The figure shows three views and two pictorial views of one solid part (mm, origin at its lowest corner). Answer the questions. A direction names the side the tool comes from. Round coordinates to 2 decimals unless told otherwise and drop trailing zeros. Order: outer loops, then holes, each group sorted by start corner. A loop starts at its lowest first (then second) coordinate and runs counter-clockwise, first axis right, second up. Notation, with made-up numbers: (77, -31) -> (97, -31) arc R20 cw to (97, -13) -> close; hole circle Ø6 at (-26.5, -36.75). An arc over 180 degrees is marked (long way). Answer in a Markdown table with one row per item. Add a question column.
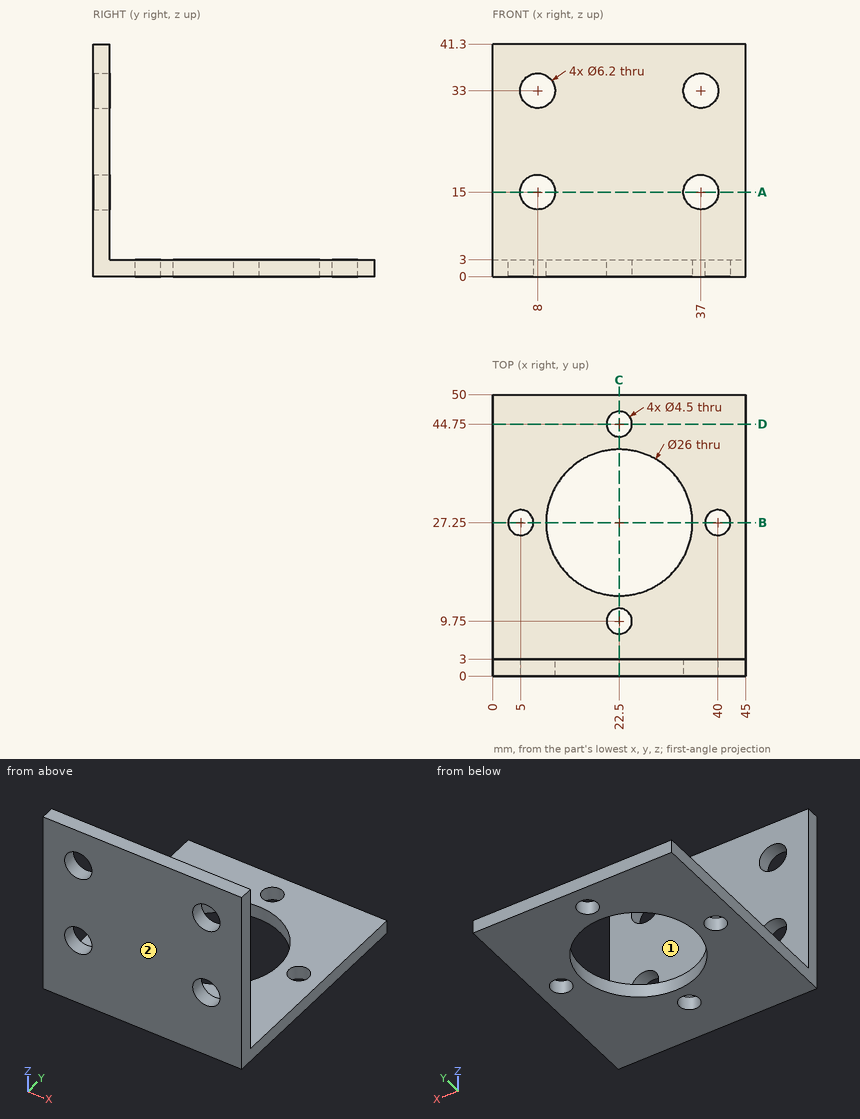
1. For the marked faces 1 and 2, determine the directions among +Z, -Z, +X, -X, +Y, -Y from which every point of the face is accessible in a straight line to the end or side of a thin tool.
2. Straight lines are drawn through the part: line 1 along Z through (x, y) = (8, 1); line 2 along X through (y, z) = (27, 2); line 3 along Y through (x, z) = (40, 1). For each, find the intervals that lie inside material, in ascending order.
3. The part is cut by section D-D (y = 44.75). Give the vertices of the cut face in (x, z).
4. The part is cut by section B-B (y = 27.25). Give the vertices of the cut face in (x, z), then the cut area to 3 significant figures.
5. The part is cut by section A-A (z = 15). Give the vertices of the cut face in (x, y).
6. Each of these flat-tipped pins is pushed along its axis until it touches: pin 1 (4 mm diameter, centred on y = 33.5, z = 5.5, fed in from -X); pin 2 (5 mm diameter, centred on x = 22.5, y = 9.75, fed in from -Z); pin 3 (19 mm diameter, centred on x = 12.5, z = 16, fed in from +Y); pin 4 (10 mm diameter, centred on x = 10, y = 43.5, fed in from +Z). Where does it stop, or does it pass through?
7. The part is cut by section C-C (x = 22.5). Give the vertices of the cut face in (y, z), then the cut area to 3 significant figures.
Report:
| question | item | result |
|---|---|---|
| 1 | face 1 | +Z, +X, -X, +Y |
| 1 | face 2 | +Z, -Z, +X, -X, -Y |
| 2 | line 1 | z = 0 to 11.9, 18.1 to 29.9, 36.1 to 41.3 |
| 2 | line 2 | x = 0 to 2.76, 7.24 to 9.5, 35.5 to 37.76, 42.24 to 45 |
| 2 | line 3 | y = 0 to 25, 29.5 to 50 |
| 3 | outline | (0, 0) -> (20.25, 0) -> (20.25, 3) -> (0, 3) -> close; (24.75, 0) -> (45, 0) -> (45, 3) -> (24.75, 3) -> close |
| 4 | outline | (0, 0) -> (2.75, 0) -> (2.75, 3) -> (0, 3) -> close; (7.25, 0) -> (9.5, 0) -> (9.5, 3) -> (7.25, 3) -> close; (35.5, 0) -> (37.75, 0) -> (37.75, 3) -> (35.5, 3) -> close; (42.25, 0) -> (45, 0) -> (45, 3) -> (42.25, 3) -> close |
| 4 | area | 30.0 mm^2 |
| 5 | outline | (0, 0) -> (4.9, 0) -> (4.9, 3) -> (0, 3) -> close; (11.1, 0) -> (33.9, 0) -> (33.9, 3) -> (11.1, 3) -> close; (40.1, 0) -> (45, 0) -> (45, 3) -> (40.1, 3) -> close |
| 6 | pin 1 | passes through |
| 6 | pin 2 | stops at z = 0 |
| 6 | pin 3 | stops at y = 3 |
| 6 | pin 4 | stops at z = 3 |
| 7 | outline | (0, 0) -> (7.5, 0) -> (7.5, 3) -> (3, 3) -> (3, 41.3) -> (0, 41.3) -> close; (12, 0) -> (14.25, 0) -> (14.25, 3) -> (12, 3) -> close; (40.25, 0) -> (42.5, 0) -> (42.5, 3) -> (40.25, 3) -> close; (47, 0) -> (50, 0) -> (50, 3) -> (47, 3) -> close |
| 7 | area | 160 mm^2 |
